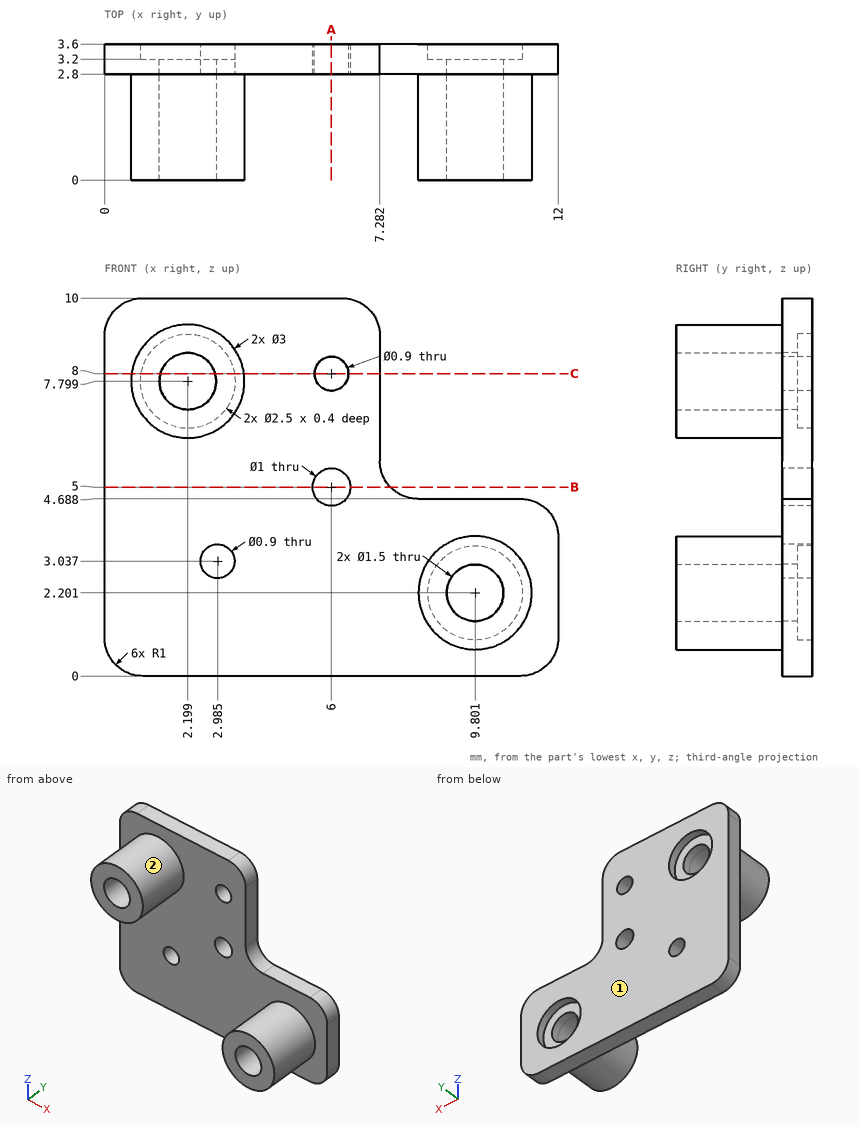
Answer from the drawing. Dimensions are ordinates in mm from the lowest x, y and z of the part. A direction names the side the tool comes from. Round coordinates to 2 decimals unless told otherwise and drop trailing zeros. Write each loop counter-clockwise with the first axis right and the second up, starting at its lowest first coordinate (ties: lowest second). Pieces come first, ordered by that corner, then holes.
1. The part is cut by section B-B, the plane z = 5. Determine the outline of the cut face in (x, y) (1 decimal).
2. Straight lines are drawn through the part: L1, parallel to Y at x = 8, z = 3.25; L2, parallel to Z at x = 2, y = 1.15 (1 decimal); L3, parallel to X at y = 0.35, z = 1.75. For each, find the intervals that lie inside material, in ascending order.
3. Given pin 1 Ø1 at (y, z) = (1.5, 8.5) entering from -X; pin 2 Ø1 at (x, y) = (1.5, 0.5) entering from -Z; pin 3 Ø2 at (x, z) = (2.2, 7.8) entering from +Y, each flat-ended and moving along its own axis, determine where each tip first touches the part or whether it passes through.
4. The part is cut by section C-C, the plane z = 8. State how many separate pieces and enclosed holes the cut face has.
5. The part is cut by section A-A, the plane x = 6. Determine the outline of the cut face in (y, z).
6. Which of the six approach directions +Z, -Z, +X, -X, +Y, -Y give full straight-line access (tool end or side, diameter ignored) to the marked faces 1 and 2?
Values:
1. outline: (0, 2.8) - (5.5, 2.8) - (5.5, 3.6) - (0, 3.6) - close; (6.5, 2.8) - (7.6, 2.8) - (7.6, 3.6) - (6.5, 3.6) - close
2. L1: y = 2.8 to 3.6
2. L2: z = 6.3 to 7.1, 8.5 to 9.3
2. L3: x = 8.37 to 9.2, 10.4 to 11.23
3. pin 1: stops at x = 0.71
3. pin 2: stops at z = 6.31
3. pin 3: stops at y = 3.2
4. separate pieces: 3
4. enclosed holes: 0
5. outline: (2.8, 0) - (3.6, 0) - (3.6, 4.5) - (2.8, 4.5) - close; (2.8, 5.5) - (3.6, 5.5) - (3.6, 7.55) - (2.8, 7.55) - close; (2.8, 8.45) - (3.6, 8.45) - (3.6, 10) - (2.8, 10) - close
6. face 1: +Z, -Z, +X, -X, +Y
6. face 2: -Y
